Solid Edge part; units mm, degrees
sketch "Sketch1" plane through (0, 0, 0) normal (0, -1, 0) x (1, 0, 0)
  line L0 (88, 26) -> (12, 26)
  line L1 (12, 26) -> (12, 12)
  line L2 (12, 12) -> (0, 12)
  line L3 (0, 12) -> (0, 0)
  line L4 (0, 0) -> (24, 0)
  line L5 (24, 0) -> (24, 10)
  line L6 (24, 10) -> (76, 10)
  line L7 (76, 10) -> (76, 0)
  line L8 (76, 0) -> (100, 0)
  line L9 (100, 0) -> (100, 12)
  line L10 (100, 12) -> (88, 12)
  line L11 (88, 12) -> (88, 26)
extrude "Protrusion1" add sketch "Sketch1" against normal blind 160
sketch "Sketch2" plane through (50, 80, 10) normal (0, 0, -1) x (1, 0, 0)
  line L0 (-6, 80) -> (-6, -50)
  line L1 (-6, -50) -> (6, -50)
  line L2 (6, -50) -> (6, 80)
  line L3 (6, 80) -> (-6, 80)
extrude "ExtrudedProtrusion_2" add sketch "Sketch2" against normal blind 72
sketch "Sketch3" plane through (88, 80, 19) normal (1, 0, 0) x (0, 1, 0)
  line L0 (80, -7) -> (80, 35)
  line L1 (20, -7) -> (80, -7)
  line L2 (20, 35) -> (20, -7)
  arc A0 (20, 35) -> (80, 35) centre (50, 35) cw
  circle A1 centre (50, 35) radius 15
extrude "ExtrudedProtrusion_3" add sketch "Sketch3" against normal blind 76
sketch "Sketch4" plane through (56, 122.5, 54) normal (1, 0, 0) x (0, 0, 1)
  arc A0 (-15, -7.5) -> (15, -7.5) centre (0, -7.5) cw
  line L0 (15, -7.5) -> (-15, -7.5)
extrude "ExtrudedCutout_1" cut sketch "Sketch4" against normal blind 12 and the other way blind 1
sketch "Sketch5" plane through (56, 59.6148, 54) normal (1, 0, 0) x (0, 1, 0)
  line L0 (-59.6148, 28) -> (59.6148, 28)
  arc A0 (50.6348, 22.5815) -> (59.6148, 28) centre (70.3852, 0) cw
  line L1 (-59.6148, -28) -> (50.6348, 22.5815)
  line L2 (-59.6148, 28) -> (-59.6148, -28)
extrude "ExtrudedCutout_3" cut sketch "Sketch5" against normal blind 12 and the other way blind 1
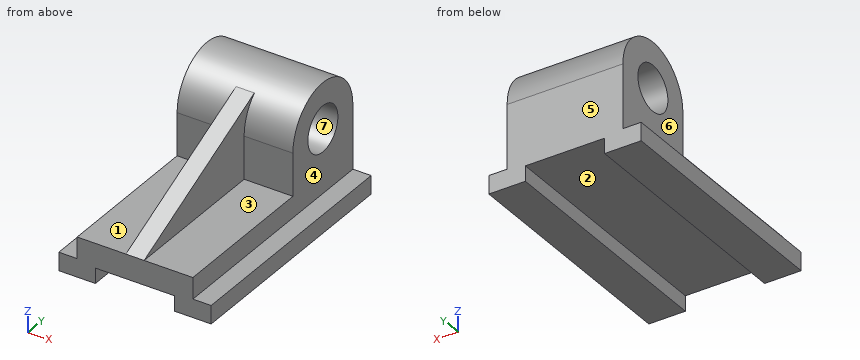
CAD build for the part. Positions are in the model's coordinates, mm. Face numbers are marked on the shaded views. A direction names the side the tool comes from. Give positions to 0.01 mm unless a question says otherwise; leave off trailing zeros. Write each loop counter-clockwise with the first axis right and the second up, starting at its lowest first coordinate (ties: lowest second). Pieces come first, ordered by that corner, then holes. Notation, with made-up numbers: (9, 53.25) - (58, 53.25) arc R28 ccw to (58, 86.25) - close; hole circle Ø5 at (20, 50). An arc over 180 degrees is marked (long way). Put each result on its own line as item: value.
(1) Saw through at D-D (y = 31). List the corners of the cut face in (x, z).
Working result:
outline: (0, 0) - (24, 0) - (24, 10) - (76, 10) - (76, 0) - (100, 0) - (100, 12) - (88, 12) - (88, 26) - (56, 26) - (56, 40.22) - (44, 40.22) - (44, 26) - (12, 26) - (12, 12) - (0, 12) - close
(2) Saw through at C-C (y = 139). List the corners of the cut face in (x, z).
Working result:
outline: (0, 0) - (24, 0) - (24, 10) - (76, 10) - (76, 0) - (100, 0) - (100, 12) - (88, 12) - (88, 42) - (12, 42) - (12, 12) - (0, 12) - close; (12, 66) - (88, 66) - (88, 82.62) - (12, 82.62) - close
(3) Saw through at A-A (x = 64.5). List the corners of the cut face in (y, z), then the cut area to 3 significant figures.
Working result:
outline: (0, 10) - (160, 10) - (160, 54) arc R30 ccw to (100, 54) - (100, 26) - (0, 26) - close; hole circle Ø30 at (130, 54)
area: 4,950 mm^2
(4) Saw through at B-B (z = 42). List the corners of the cut face in (x, y).
Working result:
outline: (12, 100) - (44, 100) - (44, 34.87) - (56, 34.87) - (56, 100) - (88, 100) - (88, 121) - (12, 121) - close; (12, 139) - (88, 139) - (88, 160) - (12, 160) - close
(5) Pull direction Y, two halves, no side cores. Call the marked faces 5, 6 and 7: released by +Y, released by -Y, zero draft, split by the parting line, or undercut.
Working result:
face 5: released by +Y
face 6: zero draft
face 7: undercut
(6) Drop flat-ended pins along their axis: pin 1 Ø8.5 at (x, z) = (79.5, 42) entering from -Y; pin 2 Ø6 at (x, y) = (38, 56) entering from -Z; pin 3 Ø1.5 at (x, z) = (36, 73.5) entering from -Y; pin 4 Ø12 at (x, z) = (39.5, 58.5) entering from +Y. Give the stop position or say it passes through.
Working result:
pin 1: y = 100
pin 2: z = 10
pin 3: y = 106.58
pin 4: y = 160
(7) Wall check: L1, parallel to Z at x = 32, y = 130; L2, parallel to Z at x = 83, y = 66.5; L3, parallel to X at y = 107.5, z = 32.5. Give the ranges that are in metal, low to high.
Working result:
L1: 10 to 39, 69 to 84
L2: 0 to 26
L3: 12 to 88
(8) Tool access for the marked faces 1, 2, 3 and 4: list every direction of +Z, -Z, +X, -X, +Y, -Y with a clear straight run to the whole face (end or side of a thin tool).
Working result:
face 1: +Z, -X, -Y
face 2: -Z, +Y, -Y
face 3: +Z, +X, -Y
face 4: +Z, +X, +Y, -Y
